Part model, mm, in its own coordinate system. A direction names the side the tool comes from. Round coordinates to 2 decimals unless told otherwise and drop trailing zeros. Loops run counter-clockwise (first coordinate to the right, second up) from the corner with the lowest first, then second, coordinate; pieces in that order, holes last.
from build123d import *

# Parameters (mm, degrees)
BOSS_EXTRUDE1_DEPTH = 10
BOSS_EXTRUDE2_START = 10
BOSS_EXTRUDE2_DEPTH = 12
BOSS_EXTRUDE3_START = 22
BOSS_EXTRUDE3_DEPTH = 12
FILLET1_R           = 10


with BuildPart() as part:
    # Sketch1 → Boss-Extrude1 (new body)
    # profile 1 of 5: a face of its own
    with BuildSketch(Plane(origin=(0, 0, 0), x_dir=(1, 0, 0), z_dir=(0, 1, 0))):
        with BuildLine():
            Line((-10, 3.266604118), (-10, -3.266604118))
            Line((-10, -3.266604118), (-6.191065945, -3.266604118))
            ThreePointArc((-6.191065945, -3.266604118), (-7, 0), (-6.191065945, 3.266604118))
            Line((-6.191065945, 3.266604118), (-10, 3.266604118))
        make_face()
    # profile 2 of 5: a face of its own
    with BuildSketch(Plane(origin=(0, 0, 0), x_dir=(1, 0, 0), z_dir=(0, 1, 0))):
        with BuildLine():
            ThreePointArc((6.191065945, 3.266604118), (0, 7), (-6.191065945, 3.266604118))
            Line((-6.191065945, 3.266604118), (6.191065945, 3.266604118))
        make_face()
    # profile 3 of 5: a face of its own
    with BuildSketch(Plane(origin=(0, 0, 0), x_dir=(1, 0, 0), z_dir=(0, 1, 0))):
        with BuildLine():
            ThreePointArc((-6.191065945, 3.266604118), (-7, 0), (-6.191065945, -3.266604118))
            Line((-6.191065945, -3.266604118), (6.191065945, -3.266604118))
            ThreePointArc((6.191065945, -3.266604118), (6.794757597, -1.68263757), (7, 0))
            ThreePointArc((7, 0), (6.794757597, 1.68263757), (6.191065945, 3.266604118))
            Line((6.191065945, 3.266604118), (-6.191065945, 3.266604118))
        make_face()
        with BuildLine():
            ThreePointArc((-1.877606485, -2.339785009), (-3, 0), (-1.877606485, 2.339785009))
            ThreePointArc((-1.877606485, 2.339785009), (1.297532378, 2.704886269), (3, 0))
            ThreePointArc((3, 0), (1.297532378, -2.704886269), (-1.877606485, -2.339785009))
        make_face(mode=Mode.SUBTRACT)
    # profile 4 of 5: a face of its own
    with BuildSketch(Plane(origin=(0, 0, 0), x_dir=(1, 0, 0), z_dir=(0, 1, 0))):
        with BuildLine():
            Line((6.191065945, -3.266604118), (-6.191065945, -3.266604118))
            ThreePointArc((-6.191065945, -3.266604118), (0, -7), (6.191065945, -3.266604118))
        make_face()
    # profile 5 of 5: a face of its own
    with BuildSketch(Plane(origin=(0, 0, 0), x_dir=(1, 0, 0), z_dir=(0, 1, 0))):
        with BuildLine():
            ThreePointArc((7, 0), (6.794757597, -1.68263757), (6.191065945, -3.266604118))
            Line((6.191065945, -3.266604118), (10, -3.266604118))
            Line((10, -3.266604118), (10, 3.266604118))
            Line((10, 3.266604118), (6.191065945, 3.266604118))
            ThreePointArc((6.191065945, 3.266604118), (6.794757597, 1.68263757), (7, 0))
        make_face()
    extrude(amount=BOSS_EXTRUDE1_DEPTH)

    # Sketch1<3> → Boss-Extrude2 (add)
    with BuildSketch(Plane(origin=(0, 0, 0), x_dir=(1, 0, 0), z_dir=(0, 1, 0)).offset(BOSS_EXTRUDE2_START)):
        with BuildLine():
            ThreePointArc((7, 0), (6.794757597, -1.68263757), (6.191065945, -3.266604118))
            Line((6.191065945, -3.266604118), (10, -3.266604118))
            Line((10, -3.266604118), (10, 3.266604118))
            Line((10, 3.266604118), (6.191065945, 3.266604118))
            ThreePointArc((6.191065945, 3.266604118), (6.794757597, 1.68263757), (7, 0))
        make_face()
        with BuildLine():
            Line((-10, 3.266604118), (-10, -3.266604118))
            Line((-10, -3.266604118), (-6.191065945, -3.266604118))
            ThreePointArc((-6.191065945, -3.266604118), (-7, 0), (-6.191065945, 3.266604118))
            Line((-6.191065945, 3.266604118), (-10, 3.266604118))
        make_face()
    extrude(amount=BOSS_EXTRUDE2_DEPTH)

    # Sketch1<5> → Boss-Extrude3 (add)
    with BuildSketch(Plane(origin=(0, 0, 0), x_dir=(1, 0, 0), z_dir=(0, 1, 0)).offset(BOSS_EXTRUDE3_START)):
        with BuildLine():
            Line((-10, 3.266604118), (-10, -3.266604118))
            Line((-10, -3.266604118), (-6.191065945, -3.266604118))
            ThreePointArc((-6.191065945, -3.266604118), (0, -7), (6.191065945, -3.266604118))
            Line((6.191065945, -3.266604118), (10, -3.266604118))
            Line((10, -3.266604118), (10, 3.266604118))
            Line((10, 3.266604118), (6.191065945, 3.266604118))
            ThreePointArc((6.191065945, 3.266604118), (0, 7), (-6.191065945, 3.266604118))
            Line((-6.191065945, 3.266604118), (-10, 3.266604118))
        make_face()
        with BuildLine():
            Line((-1.877606485, -2.339785009), (-1.877606485, 2.339785009))
            ThreePointArc((-1.877606485, 2.339785009), (3, 0), (-1.877606485, -2.339785009))
        make_face(mode=Mode.SUBTRACT)
    extrude(amount=BOSS_EXTRUDE3_DEPTH)

    # Fillet1
    # the kernel refuses this fillet: 10 mm, written as the material it adds along each edge
    with BuildSketch(Plane(origin=(6.191065945, 0, 3.266604118), x_dir=(-0.6360609802051742, 0, 0.7716387946833887), z_dir=(0, 1, 0))) as fillet1_piece_1:
        with BuildLine():
            CenterArc((4.859166888, 9.792894401), FILLET1_R, 223.265287812, 35.053552735)
            Line((-2.422714329, 2.939121283), (0, 0))
            ThreePointArc((0, 0), (1.417257009, 0.144973919), (2.834514018, 0))
        make_face()
    extrude(amount=10)
    with BuildSketch(Plane(origin=(-6.191065945, 0, 3.266604118), x_dir=(-1, 0, 0), z_dir=(0, 1, 0)), Plane(origin=(6.191065945, 0, -3.266604118), x_dir=(1, 0, 0), z_dir=(0, 1, 0))) as fillet1_piece_2:
        with BuildLine():
            CenterArc((4.465850779, 9.978399692), FILLET1_R, 231.17987933, 35.053552735)
            ThreePointArc((-1.802923765, 2.18722098), (-0.789594382, 1.185822743), (0, 0))
            Line((0, 0), (3.808934055, 0))
        make_face()
    extrude(amount=10)
    with BuildSketch(Plane(origin=(6.191065945, 22, 3.266604118), x_dir=(1, 0, 0), z_dir=(0, 1, 0))) as fillet1_piece_3:
        with BuildLine():
            CenterArc((4.465850779, -9.978399692), FILLET1_R, 93.766567935, 35.053552735)
            ThreePointArc((-1.802923765, -2.18722098), (-0.789594382, -1.185822743), (0, 0))
            Line((0, 0), (3.808934055, 0))
        make_face()
    extrude(amount=12)
    with BuildSketch(Plane(origin=(-6.191065945, 22, 3.266604118), x_dir=(-1, 0, 0), z_dir=(0, 1, 0))) as fillet1_piece_4:
        with BuildLine():
            CenterArc((4.465850779, 9.978399692), FILLET1_R, 231.17987933, 35.053552735)
            ThreePointArc((-1.802923765, 2.18722098), (-0.789594382, 1.185822743), (0, 0))
            Line((0, 0), (3.808934055, 0))
        make_face()
    extrude(amount=12)
    with BuildSketch(Plane(origin=(-6.191065945, 22, -3.266604118), x_dir=(0.6360609802051819, 0, -0.7716387946833824), z_dir=(0, 1, 0))) as fillet1_piece_5:
        with BuildLine():
            CenterArc((4.859166888, 9.792894401), FILLET1_R, 223.265287812, 35.053552735)
            Line((-2.422714329, 2.939121283), (0, 0))
            ThreePointArc((0, 0), (1.417257009, 0.144973919), (2.834514018, 0))
        make_face()
    extrude(amount=12)
    with BuildSketch(Plane(origin=(6.191065945, 22, -3.266604118), x_dir=(-0.6360609802051733, 0, -0.7716387946833895), z_dir=(0, 1, 0))) as fillet1_piece_6:
        with BuildLine():
            CenterArc((4.859166888, -9.792894401), FILLET1_R, 101.681159453, 35.053552735)
            Line((-2.422714329, -2.939121283), (0, 0))
            ThreePointArc((0, 0), (1.417257009, -0.144973919), (2.834514018, 0))
        make_face()
    extrude(amount=12)
    with BuildSketch(Plane(origin=(-6.191065945, 0, -3.266604118), x_dir=(-1, 0, 0), z_dir=(0, 1, 0))) as fillet1_piece_7:
        with BuildLine():
            CenterArc((4.465850779, -9.978399692), FILLET1_R, 93.766567935, 35.053552735)
            ThreePointArc((-1.802923765, -2.18722098), (-0.789594382, -1.185822743), (0, 0))
            Line((0, 0), (3.808934055, 0))
        make_face()
    extrude(amount=10)


solid = part.part
1) Slice it at B-B, the plane z = 2. Give the cut face in (x, y).
Values:
outline: (-10, 0) - (-2.24, 0) - (-2.24, 10) - (-6.71, 10) - (-6.71, 22) - (-1.88, 22) - (-1.88, 34) - (-10, 34) - close; (2.24, 0) - (10, 0) - (10, 34) - (2.24, 34) - (2.24, 22) - (6.71, 22) - (6.71, 10) - (2.24, 10) - close
2) Slice it at C-C, the plane y = 18. Give the cut face in (x, z), then the cut area to 3 significant figures.
Values:
outline: (-10, -3.27) - (-6.19, -3.27) arc R7 cw to (-6.19, 3.27) - (-10, 3.27) - close; (6.19, -3.27) - (10, -3.27) - (10, 3.27) - (6.19, 3.27) arc R7 cw to start
area: 42.6 mm2
3) Tool access for faces 1 (the face through (-0.1, 10, 3.2)), 2 (the face through (-8, 16, -3.267)), 3 (the face through (-1.878, 28, 0)): list every direction of +Z, -Z, +X, -X, +Y, -Y with a clear straight run to the whole face (end or side of a thin tool).
Values:
face 1: none
face 2: -Z, +X, -X
face 3: +Y, -Y
4) Slice it at D-D, the plane y = 30. Give the cut face in (x, z) (3 decimals).
Values:
outline: (-10, -3.267) arc R10 cw to (-4.388, -5.454) arc R7 ccw to (4.388, -5.454) arc R10 cw to (10, -3.267) - (10, 3.267) arc R10 cw to (4.388, 5.454) arc R7 ccw to (-4.388, 5.454) arc R10 cw to (-10, 3.267) - close; hole (-1.878, -2.34) arc R3 ccw (long way) to (-1.878, 2.34) - close
5) Drop flat-ended pins along their axis: pin 1 Ø12 at (x, y) = (8, 22) entering from -Z; pin 2 Ø1.5 at (x, y) = (3, 9) entering from -Z; pin 3 Ø1.9 at (x, y) = (8.5, 14.5) entering from +Z. Give the stop position or say it passes through.
Values:
pin 1: stops at z = -6.71
pin 2: stops at z = -6.63
pin 3: stops at z = 3.27
6) Mould opens along Y. For faces 4 (the face through (-10, 17, 0)), 5 (the face through (8, 16, 3.267)) say: released by +Y, released by -Y, zero draft, split by the parting line, or undercut.
Values:
face 4: zero draft
face 5: undercut
7) Wall check: line 1 along Y through (x, z) = (3, -0.5); line 2 along X through (y, z) = (4, 0); line 3 along Z through (x, y) = (3.25, 32). Give the ranges that are in metal, low to high.
Values:
line 1: y = 0 to 10, 22 to 34
line 2: x = -10 to -3, 3 to 10
line 3: z = -6.2 to 6.2
8) Slice it at A-A, the plane x = 0. Give the cut face in (y, z), then the cut area to 3 significant figures.
Values:
outline: (0, -7) - (10, -7) - (10, -3) - (0, -3) - close; (0, 3) - (10, 3) - (10, 7) - (0, 7) - close; (22, -7) - (34, -7) - (34, -3) - (22, -3) - close; (22, 3) - (34, 3) - (34, 7) - (22, 7) - close
area: 176 mm2
